from build123d import *

# Parameters (mm, degrees)
BOSS_EXTRUDE2_DEPTH            = 0.1
SKETCH3_R                      = 4
BOSS_EXTRUDE3_DEPTH            = 22.5
SKETCH4_R                      = 3
BOSS_EXTRUDE4_DEPTH            = 2
SKETCH5_R                      = 4
BOSS_EXTRUDE5_DEPTH            = 2
SKETCH7_W                      = 1.89865
SKETCH7_H                      = 0.1
F_6_CLEARANCE_HOLE1_AT_2_COUNT = 2
F_6_CLEARANCE_HOLE1_AT_2_PITCH = 11.930689284
F_6_32_TAPPED_HOLE1_D          = 2.7051
F_6_32_TAPPED_HOLE1_DEPTH      = 9.39
F_6_32_TAPPED_HOLE1_TIP        = 0.81269403


with BuildPart() as part:
    # Sketch2 → Boss-Extrude2 (new body)
    with BuildSketch(Plane(origin=(0, 0, 0), x_dir=(1, 0, 0), z_dir=(0, 1, 0))):
        with BuildLine():
            ThreePointArc((-1.921673483, -7.798539123), (3.967844549, -11.837003018), (9.548776015, -7.381801872))
            Line((9.548776015, -7.381801872), (10.998470019, -1.926053578))
            ThreePointArc((10.998470019, -1.926053578), (11.24988985, -0.04064778), (11.018921171, 1.84737246))
            Line((11.018921171, 1.84737246), (9.565136937, 7.567628243))
            ThreePointArc((9.565136937, 7.567628243), (3.75, 12.089730275), (-2.065136937, 7.567628243))
            Line((-2.065136937, 7.567628243), (-3.518921171, 1.84737246))
            ThreePointArc((-3.518921171, 1.84737246), (-3.749830525, -0.050419155), (-3.493426606, -1.944934706))
            Line((-3.493426606, -1.944934706), (-1.921673483, -7.798539123))
        make_face()
    extrude(amount=BOSS_EXTRUDE2_DEPTH)

    # Sketch3 → Boss-Extrude3 (add)
    with BuildSketch(Plane(origin=(0, 0.1, 0), x_dir=(1, 0, 0), z_dir=(0, 1, 0))):
        with Locations(Location((3.75, -5.840959009, 0), (0, 0, 90))):
            Circle(SKETCH3_R)
        with Locations(Location((3.75, 6.089730275, 0), (0, 0, 90))):
            Circle(SKETCH3_R)
    extrude(amount=BOSS_EXTRUDE3_DEPTH)

    # Sketch4 → Boss-Extrude4 (add)
    with BuildSketch(Plane(origin=(0, 22.6, 0), x_dir=(1, 0, 0), z_dir=(0, 1, 0))):
        with Locations(Location((3.75, -5.840959009, 0), (0, 0, 270))):
            Circle(SKETCH4_R)
        with Locations(Location((3.75, 6.089730275, 0), (0, 0, 270))):
            Circle(SKETCH4_R)
    extrude(amount=BOSS_EXTRUDE4_DEPTH)

    # Sketch5 → Boss-Extrude5 (add)
    with BuildSketch(Plane(origin=(0, 24.6, 0), x_dir=(1, 0, 0), z_dir=(0, 1, 0))):
        with Locations(Location((3.75, -5.840959009, 0), (0, 0, 90))):
            Circle(SKETCH5_R)
        with Locations(Location((3.75, 6.089730275, 0), (0, 0, 90))):
            Circle(SKETCH5_R)
    extrude(amount=BOSS_EXTRUDE5_DEPTH)

    # Sketch7 → #6 Clearance Hole1 (revolve, cut)
    with BuildSketch(Plane(origin=(3.75, 0.1, -6.089730275), x_dir=(0, 0, 1), z_dir=(1, 0, 0))):
        with Locations((0.949325, 0.05)):
            Rectangle(SKETCH7_W, SKETCH7_H)
    f_6_clearance_hole1 = revolve(axis=Axis((3.75, 6.45, -6.089730275), (0, -1, 0)), mode=Mode.SUBTRACT)

    # #6 Clearance Hole1 at 2: #6 Clearance Hole1 ×2
    with Locations(*[(0, 0, i * F_6_CLEARANCE_HOLE1_AT_2_PITCH) for i in range(1, F_6_CLEARANCE_HOLE1_AT_2_COUNT)]):
        add(f_6_clearance_hole1, mode=Mode.SUBTRACT)

    # #6-32 Tapped Hole1
    with Locations(Plane(origin=(0, 0.1, 0), x_dir=(-1, 0, 0), z_dir=(0, -1, 0))):
        with Locations((-3.75, -5.840959009), (-3.75, 6.089730275)):
            Hole(F_6_32_TAPPED_HOLE1_D / 2, depth=F_6_32_TAPPED_HOLE1_DEPTH)
            with Locations((0, 0, -(F_6_32_TAPPED_HOLE1_DEPTH + F_6_32_TAPPED_HOLE1_TIP / 2))):  # 118° drill point
                Cone(0, F_6_32_TAPPED_HOLE1_D / 2, F_6_32_TAPPED_HOLE1_TIP, mode=Mode.SUBTRACT)


solid = part.part
The model under review builds one solid part; all positions refer to its coordinate system, in mm. A direction names the side the tool comes from. Round coordinates to 2 decimals unless told otherwise and drop trailing zeros. Write each loop counter-clockwise with the first axis right and the second up, starting at its lowest first coordinate (ties: lowest second). Pieces come first, ordered by that corner, then holes. Notation, with made-up numbers: (50, -0.5) -> (94, -0.5) arc R26 cw to (94, 30.5) -> close; hole circle Ø1 at (83.5, -29). An arc over 180 degrees is marked (long way). Answer as a JSON object with one key per item and string values.
1. The part is to be moulded in two halves that separate along X. For faces 1 (the face through (1, 22.6, 4)), 2 (the face through (7.655, 11.192, 6.708)), 3 (the face through (3.781, 10.162, 5.608)), say which applies: pulls with the +X half, pulls with the -X half, needs draft (parallel to the pull), parting line crosses it, or undercut.
Results found:
{"face 1": "needs draft", "face 2": "parting line crosses it", "face 3": "undercut"}
2. We need section D-D on x = -2.5. State the section outline as (y, z) points.
Results found:
{"outline": "(0, -5.86) -> (0.1, -5.86) -> (0.1, 5.64) -> (0, 5.64) -> close"}
3. We need section A-A on z = 9.5. State the section outline as (x, y) points.
Results found:
{"outline": "(-1.01, 0) -> (8.51, 0) -> (8.51, 0.1) -> (5.37, 0.1) -> (5.37, 22.6) -> (2.13, 22.6) -> (2.13, 0.1) -> (-1.01, 0.1) -> close; (2.13, 24.6) -> (5.37, 24.6) -> (5.37, 26.6) -> (2.13, 26.6) -> close"}
4. We need section B-B on y = 20.5. State the section outline as (x, z) points.
Results found:
{"outline": "circle Ø8 at (3.75, -6.09); circle Ø8 at (3.75, 5.84)"}
5. Machinability: for faces 4 (the face through (5.282, 11.192, -9.785)), 5 (the face through (5, 0.1, 5)), 6 (the face through (1, 22.6, -8)), which of the approach directions +Z, -Z, +X, -X, +Y, -Y give a long, thin tool a straight path to every point of the face, cutting with its end or side? Answer none if there is none.
Results found:
{"face 4": "+Y", "face 5": "-Y", "face 6": "none"}
6. Clearance check with flat-ended pins moving along their axes: pin 1 (8 mm diameter, centred on y = 20, z = -4, fed in from -X); pin 2 (1.1 mm diameter, centred on x = 4.5, z = 7, fed in from -Y); pin 3 (3 mm diameter, centred on x = 3.75, z = -6.09, fed in from -Y); pin 4 (2.5 mm diameter, centred on x = 3.75, z = 5.84, fed in from -Y). State where each tip first meets the part, or that it passes through.
Results found:
{"pin 1": "stops at x = -0.25", "pin 2": "stops at y = 0", "pin 3": "stops at y = 0.1", "pin 4": "stops at y = 9.55"}
7. We need section C-C on y = 4.5. State the section outline as (x, z) points, and give its area (3 significant figures).
Results found:
{"outline": "circle Ø8 at (3.75, -6.09); circle Ø8 at (3.75, 5.84); hole circle Ø2.71 at (3.75, -6.09); hole circle Ø2.71 at (3.75, 5.84)", "area": "89.0 mm^2"}
8. To check wall thickness, follow line 1 along Z through (x, y) = (4, 7); line 2 along Y through (x, z) = (0, 5.25); line 3 along Z through (x, y) = (1, 3.5) (3 decimals). State the ranges of each line that lie inside material, in increasing order.
Results found:
{"line 1": "z = -10.08 to -7.42, -4.76 to -2.1, 1.85 to 4.51, 7.17 to 9.83", "line 2": "y = 0 to 22.6, 24.6 to 26.6", "line 3": "z = -8.994 to -3.185, 2.936 to 8.746"}
